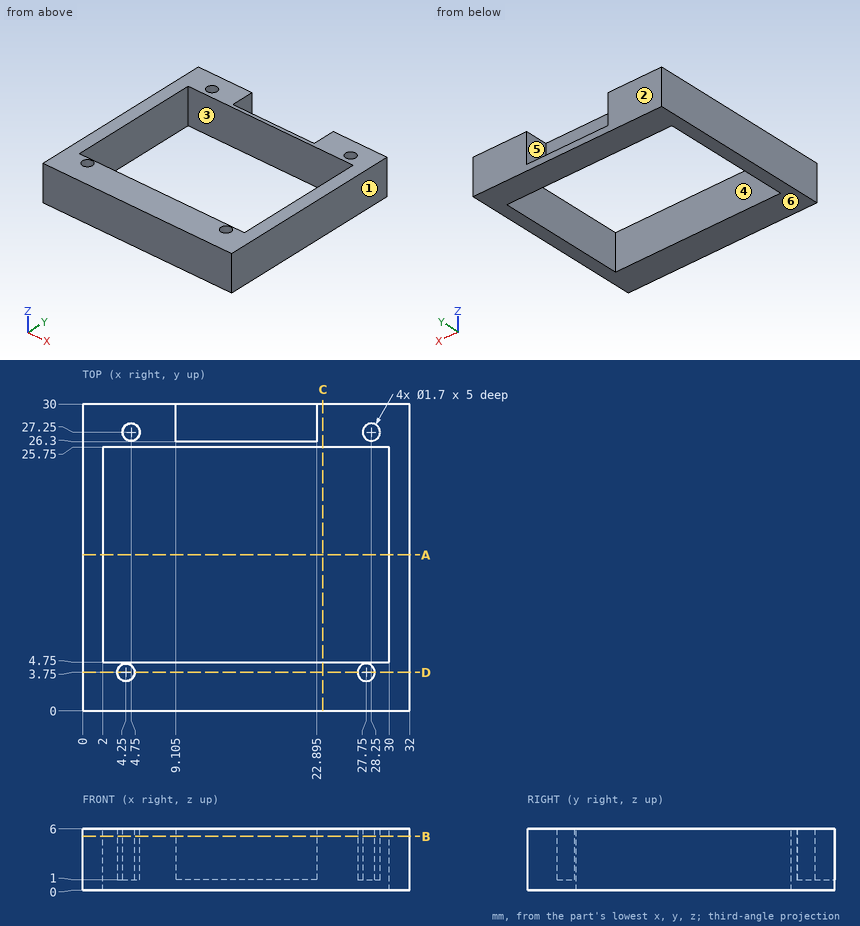
The drawing under review shows one solid part. Ordinate dimensions are in mm from its lowest x, y, z. A direction names the side the tool comes from. Round coordinates to 2 decimals unless told otherwise and drop trailing zeros. Order: outer loops, then holes, each group sorted by start corner. A loop starts at its lowest first (then second) coordinate and runs counter-clockwise, first axis right, second up. Notation, with made-up numbers: (52, 57) -> (56, 57) arc R16 cw to (56, 87) -> close; hole circle Ø8 at (-9.5, 9.25). An arc over 180 degrees is marked (long way). Return JSON: item names as keys, results as strings.
1. Take a section at B-B (z = 5.25). Write out the cut boundary in (x, y) (3 decimals).
Answer block:
{"outline": "(0, 0) -> (32, 0) -> (32, 30) -> (22.895, 30) -> (22.895, 26.3) -> (9.105, 26.3) -> (9.105, 30) -> (0, 30) -> close; hole (2, 4.75) -> (30, 4.75) -> (30, 25.75) -> (2, 25.75) -> close; hole circle Ø1.7 at (4.25, 3.75); hole circle Ø1.7 at (4.75, 27.25); hole circle Ø1.7 at (27.75, 3.75); hole circle Ø1.7 at (28.25, 27.25)"}
2. Take a section at D-D (y = 3.75). Write out the cut boundary in (x, z).
Answer block:
{"outline": "(0, 0) -> (32, 0) -> (32, 6) -> (28.6, 6) -> (28.6, 1) -> (26.9, 1) -> (26.9, 6) -> (5.1, 6) -> (5.1, 1) -> (3.4, 1) -> (3.4, 6) -> (0, 6) -> close"}
3. Insertion check: P1, Ø3, axis at y = 27.5, z = 3.5, coming from the -X side; P2, Ø0.8, axis at x = 4.5, y = 3.5, coming from the +Z side; P3, Ø1.8, axis at x = 20.5, z = 4, coming from the +Y side. Each pin has a flat end and moves straight along its axis. Give the tip position at first contact, or say it passes through.
Answer block:
{"P1": "stops at x = 0", "P2": "stops at z = 1", "P3": "stops at y = 26.3"}
4. For the marked faces 4, 5 and 6, list the 3-axis set-ups (+Z, -Z, +X, -X, +Y, -Y) from which the entire face can be reached by the end or side of a thin tool; tool diameter is ignored.
Answer block:
{"face 4": "+Z, -Z", "face 5": "+Z, +Y", "face 6": "-Z, +X, -X, +Y, -Y"}
5. Take a section at A-A (y = 15.25). Write out the cut boundary in (x, z).
Answer block:
{"outline": "(0, 0) -> (2, 0) -> (2, 6) -> (0, 6) -> close; (30, 0) -> (32, 0) -> (32, 6) -> (30, 6) -> close"}
6. For L1, parallel to X at y = 3.75, z = 3.2; L2, parallel to X at y = 27.25, z = 3.2 (3 decimals); L3, parallel to X at y = 10.5, z = 4.95, list the stretches that pass through material, from the lowest coordinate up. Write a range as [from, to].
Answer block:
{"L1": "x = [0, 3.4], [5.1, 26.9], [28.6, 32]", "L2": "x = [0, 3.9], [5.6, 9.105], [22.895, 27.4], [29.1, 32]", "L3": "x = [0, 2], [30, 32]"}
7. The part is to be moulded in two halves that separate along Y. For the marked faces 1, 2 and 3, say which applies: +Y half, -Y half, draft (parallel to the pull), parting line (faces both ways), or undercut.
Answer block:
{"face 1": "draft", "face 2": "+Y half", "face 3": "undercut"}
8. Take a section at C-C (x = 23.5). Write out the cut boundary in (y, z), then the cut area to 3 significant figures.
Answer block:
{"outline": "(0, 0) -> (4.75, 0) -> (4.75, 6) -> (0, 6) -> close; (25.75, 0) -> (30, 0) -> (30, 6) -> (25.75, 6) -> close", "area": "54.0 mm²"}
